Design review of the part built by this model. Coordinates are the model's own, in mm. A direction names the side the tool comes from. Give positions to 0.01 mm unless a question says otherwise; leave off trailing zeros. Order: outer loops, then holes, each group sorted by start corner. A loop starts at its lowest first (then second) coordinate and runs counter-clockwise, first axis right, second up.
```python
from build123d import *

# Parameters (mm, degrees)
SKETCH1_R           = 12.2
BOSS_EXTRUDE1_DEPTH = 31
SKETCH2_R           = 12.5
BOSS_EXTRUDE2_DEPTH = 21
SKETCH3_R           = 3.5
BOSS_EXTRUDE3_DEPTH = 2.5
SKETCH4_R           = 2
BOSS_EXTRUDE5_DEPTH = 1.5
BOSS_EXTRUDE6_DEPTH = 8
SKETCH6_R           = 0.5
BOSS_EXTRUDE7_DEPTH = 1
SKETCH7_R           = 7
BOSS_EXTRUDE8_DEPTH = 8


with BuildPart() as part:
    # Sketch1 → Boss-Extrude1 (new body)
    with BuildSketch(Plane.XY):
        Circle(SKETCH1_R)
    extrude(amount=BOSS_EXTRUDE1_DEPTH)

    # Sketch2 → Boss-Extrude2 (add)
    with BuildSketch(Plane.XY.offset(31)):
        with Locations(Location((0, 0, 0), (0, 0, 180))):
            Circle(SKETCH2_R)
    extrude(amount=BOSS_EXTRUDE2_DEPTH)

    # Sketch3 → Boss-Extrude3 (add)
    with BuildSketch(Plane.XY.offset(52)):
        Circle(SKETCH3_R)
    extrude(amount=BOSS_EXTRUDE3_DEPTH)

    # Sketch4 → Boss-Extrude5 (add)
    with BuildSketch(Plane.XY.offset(54.5)):
        Circle(SKETCH4_R)
    extrude(amount=BOSS_EXTRUDE5_DEPTH)

    # Sketch5 → Boss-Extrude6 (add)
    with BuildSketch(Plane.XY.offset(56)):
        with BuildLine():
            Line((0, 1.5), (1.322875656, 1.5))
            ThreePointArc((1.322875656, 1.5), (0, -2), (-1.322875656, 1.5))
            Line((-1.322875656, 1.5), (0, 1.5))
        make_face()
    extrude(amount=BOSS_EXTRUDE6_DEPTH)

    # Sketch6 → Boss-Extrude7 (add)
    with BuildSketch(Plane(origin=(0, 0, 0), x_dir=(-1, 0, 0), z_dir=(0, 0, -1))):
        with Locations(Location((0, 0, 0), (0, 0, 180))):
            Circle(SKETCH6_R)
    extrude(amount=BOSS_EXTRUDE7_DEPTH)

    # Sketch7 → Boss-Extrude8 (add)
    with BuildSketch(Plane(origin=(0, 0, -1), x_dir=(-1, 0, 0), z_dir=(0, 0, -1))):
        Circle(SKETCH7_R)
    extrude(amount=BOSS_EXTRUDE8_DEPTH)


solid = part.part
```
1. Machinability: for faces 4 (the face through (-12.19, 0.54, 15.28)), 5 (the face through (0, 1.5, 60)), 6 (the face through (-11.923, -3.755, 41.353)), 7 (the face through (3.233, -1.341, 53.232)), 8 (the face through (0, 0, 64)), which of the approach directions +Z, -Z, +X, -X, +Y, -Y give a long, thin tool a straight path to every point of the face, cutting with its end or side? Answer none if there is none.
Recorded:
face 4: -Z
face 5: +Z, +X, -X, +Y
face 6: +Z, -Z
face 7: +Z
face 8: +Z, +X, -X, +Y, -Y
2. Take a section at B-B (y = 9.75). State the section outline as (x, z) points, then the cut area to 3 significant figures.
Recorded:
outline: (-7.82, 31) - (-7.33, 31) - (-7.33, 0) - (7.33, 0) - (7.33, 31) - (7.82, 31) - (7.82, 52) - (-7.82, 52) - close
area: 783 mm2
3. For line 1 along Z through (x, y) = (1.5, 1.75); line 2 along Z through (x, y) = (-10.25, -2.75); line 3 along Z through (x, y) = (-4.5, 2.5), list the stretches that pass through material, from the lowest coordinate up.
Recorded:
line 1: z = -9 to -1, 0 to 54.5
line 2: z = 0 to 52
line 3: z = -9 to -1, 0 to 52
4. Take a section at C-C (x = 10). State the section outline as (y, z) points, then the cut area to 3 significant figures.
Recorded:
outline: (-7.5, 31) - (-6.99, 31) - (-6.99, 0) - (6.99, 0) - (6.99, 31) - (7.5, 31) - (7.5, 52) - (-7.5, 52) - close
area: 748 mm2
5. Take a section at A-A (x = -4.25). State the section outline as (y, z) points.
Recorded:
outline: (-11.76, 31) - (-11.44, 31) - (-11.44, 0) - (11.44, 0) - (11.44, 31) - (11.76, 31) - (11.76, 52) - (-11.76, 52) - close; (-5.56, -9) - (5.56, -9) - (5.56, -1) - (-5.56, -1) - close
6. For pin 1 (12 mm diameter, centred on y = 2.5, z = 19.5, fed in from +X); pin 2 (12 mm diameter, centred on y = -7.5, z = 16, fed in from -X); pin 3 (8 mm diameter, centred on y = -3, z = 10.5, fed in from -X); pin 4 (4 mm diameter, centred on x = 8.5, y = 0.5, fed in from -Z), all flat-tipped, find the tip position at first contact; note any pin that passes through.
Recorded:
pin 1: stops at x = 12.2
pin 2: stops at x = -12.11
pin 3: stops at x = -12.2
pin 4: stops at z = -9
7. Take a section at D-D (z = 38.5). State the section outline as (x, y) points.
Recorded:
outline: circle Ø25 at (0, 0)
8. Draft analysis for pull direction Z (two halves, no side actions). For faces 1 (the face through (0, 0, -9)), 2 (the face through (3, 0, 0)), 3 (the face through (-6.466, -2.681, -4.944)), state which applies: pulls with the +Z half, pulls with the -Z half, needs draft (parallel to the pull), parting line crosses it, or undercut.
Recorded:
face 1: pulls with the -Z half
face 2: undercut
face 3: needs draft
